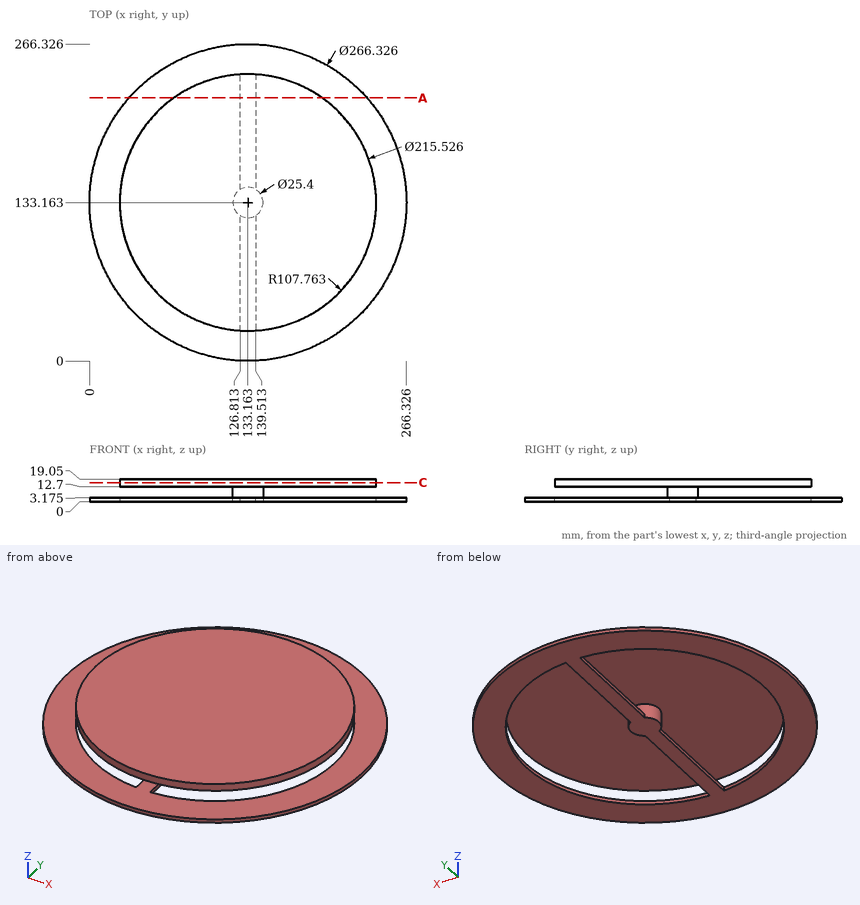
Check sheet for the drawn part. Datum: minimum x, y, z corner. Units: mm. Give positions to 0.01 mm unless a question says otherwise; leave off trailing zeros. Order: outer loops, then holes, each group sorted by start corner. A loop starts at its lowest first (then second) coordinate and runs counter-clockwise, first axis right, second up. Notation, with made-up numbers: (32, 39) -> (47, 39) arc R8 cw to (47, 45) -> close; hole circle Ø2 at (86.25, -5). An arc over 180 degrees is marked (long way). Return JSON: item names as keys, results as strings.
1. Go/stop test with flat-tipped pins: P1, Ø5, axis at x = 170.5, y = 27.5, coming from the +Z side (3 decimals); P2, Ø1, axis at x = 141.5, z = 4.5, coming from the +Y side; P3, Ø1, axis at y = 52.5, z = 1, coming from the +X side. Record where each tip stops, or that it passes through.
From the geometry:
{"P1": "z = 3.175", "P2": "y = 143.16", "P3": "x = 239.49"}
2. Cross-section at A-A, the plane y = 221. Count the separate pieces of the cut face and the enclosed holes in it, plus the area to 3 significant figures.
From the geometry:
{"separate pieces": "4", "enclosed holes": "0", "area": "1,070 mm^2"}
3. Material ranges on probe 1 along Z at (x, y) = (12, 88) (3 decimals); probe 2 along Z at (x, y) = (39, 151); probe 3 along Y at (x, z) = (126.5, 12.75), recorded low to high. Write a range as [from, to].
From the geometry:
{"probe 1": "[0, 3.175]", "probe 2": "[12.7, 19.05]", "probe 3": "[25.61, 240.72]"}
4. Cross-section at C-C, the plane z = 16. Record the cut outline in (x, y), plus the area to 3 significant figures.
From the geometry:
{"outline": "circle Ø215.53 at (133.16, 133.16)", "area": "36,500 mm^2"}
